Source: CAD feature listing. Evaluate the final solid. Frame: model axes, mm. Face numbers are marked on the shaded views. A direction names the side the tool comes from. Coordinates: 2 decimals unless noted, no trailing zeros. Loops run counter-clockwise (first coordinate to the right, second up) from the corner with the lowest first, then second, coordinate; pieces in that order, holes last. Notation, with made-up numbers: (-35.75, 78) -> (15.25, 78) arc R33 ccw to (15.25, 114) -> close; hole circle Ø5 at (-10, -36.75). An arc over 180 degrees is marked (long way). Answer as CSV lines item,"result".
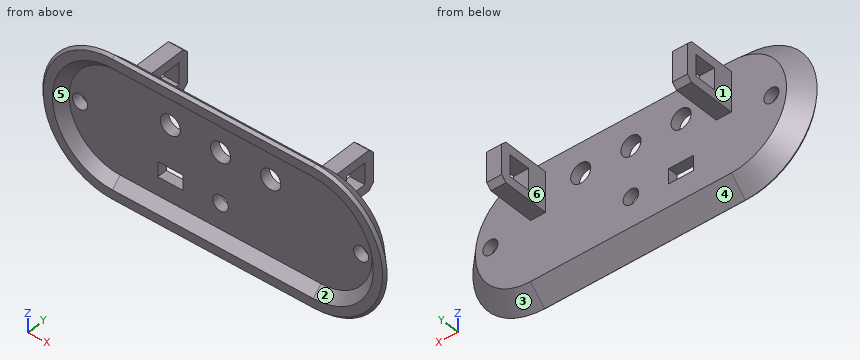
from build123d import *
from OCP.BRepFilletAPI import BRepFilletAPI_MakeChamfer

# Parameters (mm, degrees)
BOSS_EXTRU_1_DEPTH           = 3.8
BOSS_EXTRU_1_TAPER           = 45
COQUE2_DEPTH                 = 1.8
COQUE2_DRAFT                 = 45
CHANFREIN1_SIZE              = 1
CHANFREIN1_SIZE2             = 0.707106781
ENL_V_MAT_EXTRU_1_REACH      = 39.355
ESQUISSE2_R                  = 1.5
ENL_V_MAT_EXTRU_2_REACH      = 39.215
ESQUISSE3_R                  = 1.55
ESQUISSE3_R_2                = 2
ESQUISSE3_W                  = 5
ESQUISSE3_H                  = 3
ESQUISSE4_W                  = 4.3
ESQUISSE4_H                  = 4.3
BOSS_EXTRU_2_DEPTH           = 3
CHANFREIN2_SIZE              = 1
CHANFREIN2_OF_SYM_TRIE1_SIZE = 1


# Read off the part's stored shape, not the designer's step: Coque2
with BuildPart() as part:
    # Esquisse1 → Boss.-Extru.1 (new body)
    with BuildSketch(Plane(origin=(0, 0, 0), x_dir=(1, 0, 0), z_dir=(0, 1, 0))):
        with BuildLine():
            ThreePointArc((-20, 14.8), (-34.8, 0), (-20, -14.8))
            Line((-20, -14.8), (20, -14.8))
            ThreePointArc((20, -14.8), (34.8, 0), (20, 14.8))
            Line((20, 14.8), (-20, 14.8))
        make_face()
    extrude(amount=BOSS_EXTRU_1_DEPTH, taper=BOSS_EXTRU_1_TAPER)


with BuildPart() as coque2_tool:
    # Coque2 outline → Coque2 (with draft: the straight prism first)
    with BuildSketch(Plane(origin=(0, 1.8, 0), x_dir=(1, 0, 0), z_dir=(0, 1, 0))):
        with BuildLine():
            Line((-20, -10.171572875), (20, -10.171572875))
            ThreePointArc((20, -10.171572875), (30.171572875, 0), (20, 10.171572875))
            Line((20, 10.171572875), (-20, 10.171572875))
            ThreePointArc((-20, 10.171572875), (-30.171572875, 0), (-20, -10.171572875))
        make_face()
    extrude(amount=-COQUE2_DEPTH)
    # Coque2: the draft: its side faces are tilted about the plane it starts from
    coque2_sides = [coque2_tool.faces().sort_by_distance(p)[0] for p in [
        (0, 0.9, 10.171572875),
        (30.171572875, 0.9, 0),
        (0, 0.9, -10.171572875),
        (-30.171572875, 0.9, 0),
    ]]
    draft(coque2_sides, Plane(origin=(0, 1.8, 0), x_dir=(1, 0, 0), z_dir=(0, 1, 0)), COQUE2_DRAFT)


with BuildPart() as part_1:
    add(part.part)

    # Coque2: cut by coque2_tool
    add(coque2_tool.part, mode=Mode.SUBTRACT)

    # Chanfrein1: one chamfer whose edges measure the first distance from different faces: ONE call of the kernel's chamfer builder (chamfer() names one face for all edges)
    chanfrein1_edges_1 = [part_1.edges().sort_by_distance(p)[0] for p in [
        (0, 0, -14.8),
        (0, 0, 14.8),
        (-34.8, 0, 0),
    ]]
    chanfrein1_side_1 = [part_1.faces().sort_by_distance(p)[0] for p in [
        (0, 0, -14.043672029),
    ]]
    chanfrein1_edges_2 = [part_1.edges().sort_by_distance(p)[0] for p in [
        (34.8, 0, 0),
    ]]
    chanfrein1_side_2 = [part_1.faces().sort_by_distance(p)[0] for p in [
        (32.9, 1.9, 0),
    ]]
    chanfrein1 = BRepFilletAPI_MakeChamfer(part_1.part.solid().wrapped)
    for e in chanfrein1_edges_1:
        chanfrein1.Add(CHANFREIN1_SIZE, CHANFREIN1_SIZE2, e.wrapped, chanfrein1_side_1[0].wrapped)  # the first distance lies on this face
    for e in chanfrein1_edges_2:
        chanfrein1.Add(CHANFREIN1_SIZE, CHANFREIN1_SIZE2, e.wrapped, chanfrein1_side_2[0].wrapped)  # the first distance lies on this face
    add(Compound.cast(chanfrein1.Shape()), mode=Mode.REPLACE)

    # Esquisse2 → Enlèv. mat.-Extru.1 (cut, up to next)
    with BuildSketch(Plane(origin=(0, 3.8, 0), x_dir=(1, 0, 0), z_dir=(0, 1, 0)), mode=Mode.PRIVATE) as enl_v_mat_extru_1_sk1:
        with Locations(Location((-28, 0, 0), (0, 0, 270))):
            Circle(ESQUISSE2_R)
    enl_v_mat_extru_1_tool1 = extrude(enl_v_mat_extru_1_sk1.sketch, amount=-ENL_V_MAT_EXTRU_1_REACH, mode=Mode.PRIVATE) & part_1.part
    # Esquisse2 → Enlèv. mat.-Extru.1 (cut, up to next)
    with BuildSketch(Plane(origin=(0, 3.8, 0), x_dir=(1, 0, 0), z_dir=(0, 1, 0)), mode=Mode.PRIVATE) as enl_v_mat_extru_1_sk2:
        with Locations(Location((28, 0, 0), (0, 0, 270))):
            Circle(ESQUISSE2_R)
    enl_v_mat_extru_1_tool2 = extrude(enl_v_mat_extru_1_sk2.sketch, amount=-ENL_V_MAT_EXTRU_1_REACH, mode=Mode.PRIVATE) & part_1.part
    add(enl_v_mat_extru_1_tool1.solids().sort_by_distance((-28, 3.8, 0))[0], mode=Mode.SUBTRACT)
    add(enl_v_mat_extru_1_tool2.solids().sort_by_distance((28, 3.8, 0))[0], mode=Mode.SUBTRACT)

    # Esquisse3 → Enlèv. mat.-Extru.2 (cut, up to next)
    with BuildSketch(Plane.XZ.offset(-1.8), mode=Mode.PRIVATE) as enl_v_mat_extru_2_sk1:
        with Locations(Location((0, -5, 0), (0, 0, 270))):
            Circle(ESQUISSE3_R)
    enl_v_mat_extru_2_tool1 = extrude(enl_v_mat_extru_2_sk1.sketch, amount=-ENL_V_MAT_EXTRU_2_REACH, mode=Mode.PRIVATE) & part_1.part
    # Esquisse3 → Enlèv. mat.-Extru.2 (cut, up to next)
    with BuildSketch(Plane.XZ.offset(-1.8), mode=Mode.PRIVATE) as enl_v_mat_extru_2_sk2:
        with Locations(Location((10, 5, 0), (0, 0, 270))):
            Circle(ESQUISSE3_R_2)
    enl_v_mat_extru_2_tool2 = extrude(enl_v_mat_extru_2_sk2.sketch, amount=-ENL_V_MAT_EXTRU_2_REACH, mode=Mode.PRIVATE) & part_1.part
    # Esquisse3 → Enlèv. mat.-Extru.2 (cut, up to next)
    with BuildSketch(Plane.XZ.offset(-1.8), mode=Mode.PRIVATE) as enl_v_mat_extru_2_sk3:
        with Locations(Location((0, 5, 0), (0, 0, 270))):
            Circle(ESQUISSE3_R_2)
    enl_v_mat_extru_2_tool3 = extrude(enl_v_mat_extru_2_sk3.sketch, amount=-ENL_V_MAT_EXTRU_2_REACH, mode=Mode.PRIVATE) & part_1.part
    # Esquisse3 → Enlèv. mat.-Extru.2 (cut, up to next)
    with BuildSketch(Plane.XZ.offset(-1.8), mode=Mode.PRIVATE) as enl_v_mat_extru_2_sk4:
        with Locations(Location((-10, 5, 0), (0, 0, 270))):
            Circle(ESQUISSE3_R_2)
    enl_v_mat_extru_2_tool4 = extrude(enl_v_mat_extru_2_sk4.sketch, amount=-ENL_V_MAT_EXTRU_2_REACH, mode=Mode.PRIVATE) & part_1.part
    # Esquisse3 → Enlèv. mat.-Extru.2 (cut, up to next)
    with BuildSketch(Plane.XZ.offset(-1.8), mode=Mode.PRIVATE) as enl_v_mat_extru_2_sk5:
        with Locations((-10, -5)):
            Rectangle(ESQUISSE3_W, ESQUISSE3_H)
    enl_v_mat_extru_2_tool5 = extrude(enl_v_mat_extru_2_sk5.sketch, amount=-ENL_V_MAT_EXTRU_2_REACH, mode=Mode.PRIVATE) & part_1.part
    add(enl_v_mat_extru_2_tool1.solids().sort_by_distance((0, 1.8, -5))[0], mode=Mode.SUBTRACT)
    add(enl_v_mat_extru_2_tool2.solids().sort_by_distance((10, 1.8, 5))[0], mode=Mode.SUBTRACT)
    add(enl_v_mat_extru_2_tool3.solids().sort_by_distance((0, 1.8, 5))[0], mode=Mode.SUBTRACT)
    add(enl_v_mat_extru_2_tool4.solids().sort_by_distance((-10, 1.8, 5))[0], mode=Mode.SUBTRACT)
    add(enl_v_mat_extru_2_tool5.solids().sort_by_distance((-10, 1.8, -5))[0], mode=Mode.SUBTRACT)

    # Esquisse4 → Boss.-Extru.2 (add)
    with BuildSketch(Plane.ZY.offset(-20)):
        Polygon((9, 3.8), (1, 3.8), (1, 14.1), (5, 14.1), (9, 14.1), align=None)
        with Locations((5, 9.95)):
            Rectangle(ESQUISSE4_W, ESQUISSE4_H, mode=Mode.SUBTRACT)
    boss_extru_2 = extrude(amount=BOSS_EXTRU_2_DEPTH)

    # Chanfrein2
    chanfrein2_edges = [part_1.edges().sort_by_distance(p)[0] for p in [
        (18.5, 14.1, 9),
        (18.5, 14.1, 1),
    ]]
    chamfer(chanfrein2_edges, length=CHANFREIN2_SIZE)

    # Symétrie1: Boss.-Extru.2 across plane
    add(boss_extru_2.mirror(Plane(origin=(0, 0, 0), x_dir=(0, 0, 1), z_dir=(1, 0, 0))))

    # Chanfrein2 of Symétrie1
    chanfrein2_of_sym_trie1_edges = [part_1.edges().sort_by_distance(p)[0] for p in [
        (-18.5, 14.1, 9),
        (-18.5, 14.1, 1),
    ]]
    chamfer(chanfrein2_of_sym_trie1_edges, length=CHANFREIN2_OF_SYM_TRIE1_SIZE)


solid = part_1.part
(1) Material intervals for L1, parallel to X at y = 3, z = -0.5; L2, parallel to X at y = 8.5, z = 2.5; L3, parallel to Y at x = 20.5, z = 5, sorted ascending. Write a range as [from, to].
Computed values:
L1,"[-31.79, -29.41], [-26.59, 26.59], [29.41, 31.79]"
L2,"[-20, -17], [17, 20]"
L3,"[1.8, 3.8]"
(2) Cut plane A-A (y = 10). Return the cut outline in (x, z).
Computed values:
outline,"(-20, 1) -> (-17, 1) -> (-17, 2.85) -> (-20, 2.85) -> close; (-20, 7.15) -> (-17, 7.15) -> (-17, 9) -> (-20, 9) -> close; (17, 1) -> (20, 1) -> (20, 2.85) -> (17, 2.85) -> close; (17, 7.15) -> (20, 7.15) -> (20, 9) -> (17, 9) -> close"
(3) Access query for the marked faces 4, 5 and 6. Directions: +Z, -Z, +X, -X, +Y, -Y. A direction counts if a zero-diameter tool reaches every point of the face in a straight line with its end or side. Return the directions, or none.
Computed values:
face 4,"-Z, +X, -X, +Y"
face 5,"-Y"
face 6,"+Z, -Z, +Y"
(4) Draft query along X for the marked faces 1, 2 and 3. Return one class per face: released by +X, released by -X, zero draft, split by the parting line, or undercut.
Computed values:
face 1,"released by -X"
face 2,"undercut"
face 3,"released by +X"
(5) Cut plane B-B (x = -10). Return the cut outline in (y, z).
Computed values:
outline,"(0, -13.8) -> (0.5, -14.3) -> (3.8, -11) -> (3.8, -6.5) -> (1.8, -6.5) -> (1.8, -10.17) -> (0, -11.97) -> close; (0, 11.97) -> (1.8, 10.17) -> (1.8, 7) -> (3.8, 7) -> (3.8, 11) -> (0.5, 14.3) -> (0, 13.8) -> close; (1.8, -3.5) -> (3.8, -3.5) -> (3.8, 3) -> (1.8, 3) -> close"
(6) Pin query (flat end, axial travel): pin 1 Ø3.5 at (x, z) = (0, -5) entering from -Y; pin 2 Ø2.5 at (x, y) = (19, 9.5) entering from +Z; pin 3 Ø4.5 at (x, z) = (10, 5) entering from +Y. Return the tip coordinate at first contact, or that it passes through.
Computed values:
pin 1,"y = 1.8"
pin 2,"z = 9"
pin 3,"y = 3.8"
(7) Cut plane D-D (y = 5.5). Return the cut outline in (x, z).
Computed values:
outline,"(-20, 1) -> (-17, 1) -> (-17, 9) -> (-20, 9) -> close; (17, 1) -> (20, 1) -> (20, 9) -> (17, 9) -> close"
(8) Cut plane C-C (z = 0). Return the cut outline in (x, y).
Computed values:
outline,"(-34.3, 0.5) -> (-33.8, 0) -> (-31.97, 0) -> (-30.17, 1.8) -> (-29.5, 1.8) -> (-29.5, 3.8) -> (-31, 3.8) -> close; (-26.5, 1.8) -> (26.5, 1.8) -> (26.5, 3.8) -> (-26.5, 3.8) -> close; (29.5, 1.8) -> (30.17, 1.8) -> (31.97, 0) -> (33.8, 0) -> (34.3, 0.5) -> (31, 3.8) -> (29.5, 3.8) -> close"
